```python
from build123d import *

# Parameters (mm, degrees)
F0_W     = 19.05
F0_H     = 19.05
F1_DEPTH = 19.05
F3_DEPTH = 12.7
F5_DEPTH = 19.05
F6_DEPTH = 12.7


with BuildPart() as f1:
    # F0 (on Top) → F1 (new body)
    with BuildSketch(Plane.XY):
        with Locations((9.525, 9.525)):
            Rectangle(F0_W, F0_H)
    extrude(amount=F1_DEPTH)

    # F2 (on face) → F3 (cut)
    with BuildSketch(Plane.YZ.offset(19.05)):
        Polygon((4.7625, 15.875), (3.175, 15.875), (3.175, 3.175), (15.875, 3.175), (15.875, 4.7625), (4.7625, 4.7625), align=None)
    extrude(amount=-F3_DEPTH, mode=Mode.SUBTRACT)

    # F4 (on face) → F5 (join)
    with BuildSketch(Plane.YZ.offset(19.05)):
        Polygon((2.7797596434, 34.8148003284), (0, 19.05), (19.05, 19.05), (21.2553318564, 31.5570584633), align=None)
    extrude(amount=-F5_DEPTH)

    # F6 (add): a face of the model
    f6_faces = [f1.faces().sort_by_distance(p)[0] for p in [
        (9.525, 19.05, 9.525),
    ]]
    extrude(f6_faces, amount=F6_DEPTH)


solid = f1.part
```
Model file for the job. Use its own axes, mm. A direction names the side the tool comes from. Coordinates: 2 decimals unless noted, no trailing zeros. Order: outer loops, then holes, each group sorted by start corner. A loop starts at its lowest first (then second) coordinate and runs counter-clockwise, first axis right, second up. Notation, with made-up numbers: (44.25, 52.5) -> (62.25, 52.5) arc R18 ccw to (62.25, 73.5) -> close; hole circle Ø11 at (76.5, 68.25). An arc over 180 degrees is marked (long way). Answer as a JSON object with one key per item and string values. Group by question number.
1) Drill centre lines: L1, parallel to Z at x = 8.5, y = 8 (1 decimal); L2, parallel to Z at x = 8, y = 27.5; L3, parallel to Z at x = 18, y = 6.5 (1 decimal). Where is each one in solid material? Low to high.
2) Which spindle directions (+Z, -Z, +X, -X, +Y, -Y) get a long thin tool onto all of the face, cutting with end or side? Do faces 5 (the face through (13, 4, 15.875)), 6 (the face through (9, 25, 19.05)), 7 (the face through (9, 31.75, 9)). Say none if no direction does.
3) Flat gauge pins, fed straight in: pin 1 (6 mm diameter, centred on x = 13, y = 6, fed in from +Z); pin 2 (1 mm diameter, centred on x = 3.5, z = 29.5, fed in from +Y); pin 3 (6.5 mm diameter, centred on x = 10, y = 8, fed in from +Z). Where does each tip first touch, or does it go through?
4) Cut at D-D, the plane y = 25.5. Write the cut outline in (x, z).
5) Pull direction Z, two halves, no side cores. Call faces 1 (the face through (13, 4.762, 10)), 2 (the face through (6.35, 7, 4)), 3 (the face through (9, 0, 9)), 4 (the face through (9, 16, 0)): +Z half, -Z half, draft (parallel to the pull), parting line (faces both ways), or undercut.
Check values:
{
 "1": {"L1": "z = 0 to 3.2, 4.8 to 33.9", "L2": "z = 0 to 19.05", "L3": "z = 0 to 3.2, 4.8 to 34.2"},
 "2": {"face 5": "+X", "face 6": "+X, -X, +Y", "face 7": "+Z, -Z, +X, -X, +Y"},
 "3": {"pin 1": "stops at z = 34.78", "pin 2": "stops at y = 20.98", "pin 3": "stops at z = 34.47"},
 "4": {"outline": "(0, 0) -> (19.05, 0) -> (19.05, 19.05) -> (0, 19.05) -> close"},
 "5": {"face 1": "undercut", "face 2": "undercut", "face 3": "draft", "face 4": "-Z half"}
}
